from build123d import *

# Parameters (mm, degrees)
CROQUIS1_W              = 8
CROQUIS1_H              = 8
CROQUIS1_R              = 1
CROQUIS1_W_2            = 10
CROQUIS1_H_2            = 3
CROQUIS1_W_3            = 3
CROQUIS1_H_3            = 10
SALIENTE_EXTRUIR1_DEPTH = 3
CROQUIS2_W              = 114
CROQUIS2_H              = 8
CORTAR_EXTRUIR1_DEPTH   = 4
CROQUIS3_W              = 114
CROQUIS3_H              = 2
CORTAR_EXTRUIR2_DEPTH   = 4


with BuildPart() as part:
    # Croquis1 → Saliente-Extruir1 (new body)
    with BuildSketch(Plane(origin=(0, 0, 0), x_dir=(1, 0, 0), z_dir=(0, 1, 0))):
        Polygon((-57, 0), (-57, -15), (-38, -15), (-38, -45), (-57, -45), (-57, -50), (-60, -50), (-60, -55), (-57, -55), (-57, -60), (57, -60), (57, -55), (60, -55), (60, -50), (57, -50), (57, -45), (38, -45), (38, -15), (57, -15), (57, 0), (60, 0), (60, 15), (57, 15), (57, 30), (60, 30), (60, 45), (57, 45), (57, 60), (-57, 60), (-57, 45), (-60, 45), (-60, 30), (-57, 30), (-57, 15), (-60, 15), (-60, 0), align=None)
        with Locations((-45, -51.5)):
            Rectangle(CROQUIS1_W, CROQUIS1_H, mode=Mode.SUBTRACT)
        with Locations((-24.95, -39)):
            Circle(CROQUIS1_R, mode=Mode.SUBTRACT)
        with Locations((-24.95, -21)):
            Circle(CROQUIS1_R, mode=Mode.SUBTRACT)
        with Locations((-20, -7)):
            Circle(CROQUIS1_R, mode=Mode.SUBTRACT)
        with Locations((24.95, -39)):
            Circle(CROQUIS1_R, mode=Mode.SUBTRACT)
        with Locations((45, -51.5)):
            Rectangle(CROQUIS1_W, CROQUIS1_H, mode=Mode.SUBTRACT)
        with Locations((24.95, -21)):
            Circle(CROQUIS1_R, mode=Mode.SUBTRACT)
        with Locations((0, -7)):
            Rectangle(CROQUIS1_W_2, CROQUIS1_H_2, mode=Mode.SUBTRACT)
        with Locations((20, -7)):
            Circle(CROQUIS1_R, mode=Mode.SUBTRACT)
        with Locations((-36.5, 12)):
            Rectangle(CROQUIS1_W_3, CROQUIS1_H_3, mode=Mode.SUBTRACT)
        with Locations((-43, 44)):
            Rectangle(CROQUIS1_W, CROQUIS1_H, mode=Mode.SUBTRACT)
        with Locations((-20, 31)):
            Circle(CROQUIS1_R, mode=Mode.SUBTRACT)
        with Locations((36.5, 12)):
            Rectangle(CROQUIS1_W_3, CROQUIS1_H_3, mode=Mode.SUBTRACT)
        with Locations((0, 31)):
            Rectangle(CROQUIS1_W_2, CROQUIS1_H_2, mode=Mode.SUBTRACT)
        with Locations((20, 31)):
            Circle(CROQUIS1_R, mode=Mode.SUBTRACT)
        with Locations((43, 44)):
            Rectangle(CROQUIS1_W, CROQUIS1_H, mode=Mode.SUBTRACT)
    extrude(amount=SALIENTE_EXTRUIR1_DEPTH)

    # Croquis2 → Cortar-Extruir1 (cut, through all)
    with BuildSketch(Plane(origin=(0, 3, 0), x_dir=(1, 0, 0), z_dir=(0, 1, 0))):
        with Locations((0, 56)):
            Rectangle(CROQUIS2_W, CROQUIS2_H)
    extrude(amount=-CORTAR_EXTRUIR1_DEPTH, mode=Mode.SUBTRACT)

    # Croquis3 → Cortar-Extruir2 (cut, through all)
    with BuildSketch(Plane(origin=(0, 3, 0), x_dir=(1, 0, 0), z_dir=(0, 1, 0))):
        with Locations((0, -59)):
            Rectangle(CROQUIS3_W, CROQUIS3_H)
    extrude(amount=-CORTAR_EXTRUIR2_DEPTH, mode=Mode.SUBTRACT)


solid = part.part
Here's how the part is built. I have some questions about the finished solid (model axes, mm). A direction names the side the tool comes from. Give positions to 0.01 mm unless a question says otherwise; leave off trailing zeros. Order: outer loops, then holes, each group sorted by start corner. A loop starts at its lowest first (then second) coordinate and runs counter-clockwise, first axis right, second up. Notation, with made-up numbers: M 28.25,-7.5 L 60.25,-7.5 A16 cw 60.25,9.5 Z; hole C 38.5,-8 d10. An arc over 180 degrees is marked long. Answer as a JSON object with one key per item and string values. Group by question number.
1) We'd pull the mould along X, two halves only. Please class faces 1 (the flat face through (-60, 1, -8)), 2 (the flat face through (41, 1, 52)), 3 (the flat face through (35, 1, -12)), 4 (the flat face through (-58, 1, 50)): pulls with the +X half, pulls with the -X half, needs draft (parallel to the pull), parting line crosses it, or undercut.
2) I'm going to push flat-ended pins straight in: pin 1 Ø0.9 at (x, y) = (-58.5, 1) entering from +Z; pin 2 Ø1.6 at (x, z) = (-24.95, 21) entering from -Y; pin 3 Ø0.9 at (y, z) = (1, -46) entering from +X; pin 4 Ø1.5 at (y, z) = (1.5, 57) entering from -X. Where does each tip first touch, or does it pass through?
3) Suppose I cut it at C-C, the plane z = 24. Write out the boundary of the cut face in (x, y), plus the area to 3 significant figures.
4) Suppose I cut it at B-B, the plane y = 0.8. Count the separate pieces of the cut face and the enclosed holes in it, plus the area to 3 significant figures.
5) Please list where these lines run through material, in increasing order: L1, parallel to Z at x = 20, y = 1.95; L2, parallel to X at y = 1.8, z = -12.5; L3, parallel to Z at x = 24.95, y = 1.2. Write a range as [from, to].
6) Suppose I cut it at A-A, the plane x = -50.5. Write out the boundary of the cut face in (y, z), plus the area to 3 significant figures.
7) On a 3-axis mill with a long thin cutter (end or side, diameter ignored), from which of +Z, -Z, +X, -X, +Y, -Y can I reach the whole of each face in a straight line? I mean faces 5 (the flat face through (57, 1, -22)), 6 (the flat face through (39, 1, -44)), 7 (the flat face through (57, 1, 57)), 8 (the flat face through (-57, 1, 7)). Say none if no direction works.
Results found:
{
 "1": {"face 1": "pulls with the -X half", "face 2": "undercut", "face 3": "undercut", "face 4": "needs draft"},
 "2": {"pin 1": "z = 55", "pin 2": "through", "pin 3": "x = 57", "pin 4": "x = -57"},
 "3": {"outline": "M -38,0 L 38,0 L 38,3 L -38,3 Z", "area": "228 mm²"},
 "4": {"separate pieces": "1", "enclosed holes": "16", "area": "11,200 mm²"},
 "5": {"L1": "[-52, -32], [-30, 6], [8, 58]", "L2": "[-60, -38], [-35, 35], [38, 60]", "L3": "[-52, 20], [22, 38], [40, 58]"},
 "6": {"outline": "M 0,-52 L 3,-52 L 3,15 L 0,15 Z; M 0,45 L 3,45 L 3,58 L 0,58 Z", "area": "240 mm²"},
 "7": {"face 5": "+X, +Y, -Y", "face 6": "+Y, -Y", "face 7": "+Z, +X, +Y, -Y", "face 8": "-X, +Y, -Y"}
}
